Design review of the part shown in the three views and the two pictorial views. Dimensions are in mm from the part's minimum x, y and z. A direction names the side the tool comes from. Give positions to 0.01 mm unless a question says otherwise; leave off trailing zeros. Write each loop counter-clockwise with the first axis right and the second up, starting at its lowest first coordinate (ties: lowest second). Pieces come first, ordered by that corner, then holes. Notation, with made-up numbers: (12, 88) -> (63, 88) arc R29 ccw to (63, 121) -> close; hole circle Ø2 at (6, 16). An arc over 180 degrees is marked (long way). Return JSON: item names as keys, results as strings. Group by question number.
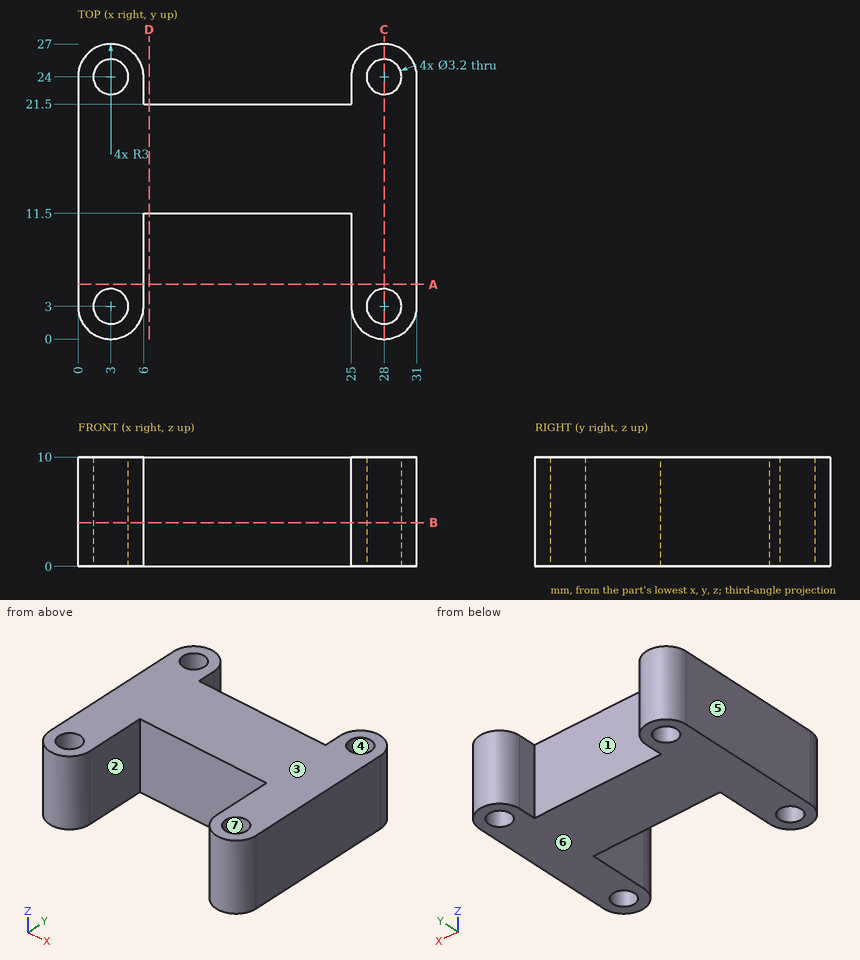
Q1. Mouldability with a two-part tool opening along X and no side actions: class the marked faces 4, 5, 6 and 7 as +X half, -X half, draft (parallel to the pull), parting line (faces both ways), or undercut.
Q2. Take a section at B-B, the plane z = 4. Give the boundary of the cut face in (x, y).
Q3. Take a section at A-A, the plane y = 5. Give the boundary of the cut face in (x, z), plus the area to 3 significant figures.
Q4. Take a section at C-C, the plane x = 28. Give the boundary of the cut face in (y, z), plus the area to 3 significant figures.
Q5. Insertion check: pin 1 (3 mm diameter, centred on x = 28, y = 24, fed in from +Z); pin 2 (5 mm diameter, centred on x = 17, z = 6.5, fed in from -Y); pin 3 (3 mm diameter, centred on x = 15.5, z = 7, fed in from +Y); pin 4 (3 mm diameter, centred on x = 25.5, z = 9, fed in from +Y). Each pin has a flat end and moves straight along its axis. Give the tip position at first contact, or say it passes through.
Q6. For L1, parallel to Y at x = 28, z = 6.75; L2, parallel to X at y = 25, z = 5.5; L3, parallel to X at y = 2.75, z = 1.25, list the stretches that pass through material, from the lowest coordinate up. Write a range as from..to.
Q7. Tool access review of the marked faces 1, 2 and 3: name each direction out of +Z, -Z, +X, -X, +Y, -Y from which nothing blocks a thin tool from reaching the whole face with its end or side.
Q8. Take a section at D-D, the plane x = 6.5. Give the boundary of the cut face in (y, z), plus the area to 3 significant figures.
Final values:
{
 "1": {"face 4": "undercut", "face 5": "-X half", "face 6": "draft", "face 7": "undercut"},
 "2": {"outline": "(0, 3) arc R3 ccw to (6, 3) -> (6, 11.5) -> (25, 11.5) -> (25, 3) arc R3 ccw to (31, 3) -> (31, 24) arc R3 ccw to (25, 24) -> (25, 21.5) -> (6, 21.5) -> (6, 24) arc R3 ccw to (0, 24) -> close; hole circle Ø3.2 at (3, 3); hole circle Ø3.2 at (3, 24); hole circle Ø3.2 at (28, 3); hole circle Ø3.2 at (28, 24)"},
 "3": {"outline": "(0, 0) -> (6, 0) -> (6, 10) -> (0, 10) -> close; (25, 0) -> (31, 0) -> (31, 10) -> (25, 10) -> close", "area": "120 mm²"},
 "4": {"outline": "(0, 0) -> (1.4, 0) -> (1.4, 10) -> (0, 10) -> close; (4.6, 0) -> (22.4, 0) -> (22.4, 10) -> (4.6, 10) -> close; (25.6, 0) -> (27, 0) -> (27, 10) -> (25.6, 10) -> close", "area": "206 mm²"},
 "5": {"pin 1": "passes through", "pin 2": "stops at y = 11.5", "pin 3": "stops at y = 21.5", "pin 4": "stops at y = 26.83"},
 "6": {"L1": "y = 0..1.4, 4.6..22.4, 25.6..27", "L2": "x = 0.17..1.75, 4.25..5.83, 25.17..26.75, 29.25..30.83", "L3": "x = 0.01..1.42, 4.58..5.99, 25.01..26.42, 29.58..30.99"},
 "7": {"face 1": "+Z, -Z, +Y", "face 2": "+Z, -Z, -Y", "face 3": "+Z, +X, -X, +Y, -Y"},
 "8": {"outline": "(11.5, 0) -> (21.5, 0) -> (21.5, 10) -> (11.5, 10) -> close", "area": "100 mm²"}
}
